CAD build for the part. Positions are in the model's coordinates, mm. A direction names the side the tool comes from. Round coordinates to 2 decimals unless told otherwise and drop trailing zeros. Order: outer loops, then holes, each group sorted by start corner. A loop starts at its lowest first (then second) coordinate and runs counter-clockwise, first axis right, second up. Notation, with made-up numbers: (26, 37) -> (47, 37) arc R32 cw to (47, 70) -> close; hole circle Ø9 at (-32.75, 1.5). An arc over 180 degrees is marked (long way). Return JSON: item names as keys, results as strings. Group by question number.
Q1. Which spindle directions (+Z, -Z, +X, -X, +Y, -Y) get a long thin tool onto all of the face, cutting with end or side? Do faces 4 (the flat face through (10, -0.574, 2)), 5 (the cylindrical face through (7.214, 13.802, 0.493)), 6 (the cylindrical face through (0.07, -2.96, 2.99)), 7 (the flat face through (-15, 22, 0)). Say none if no direction does.
Q2. Flat gauge pins, fed straight in: pin 1 (0.5 mm diameter, centred on y = 7, z = 3, fed in from +X); pin 2 (12.5 mm diameter, centred on x = 7, y = 3.5, fed in from +Z). Where does each tip first touch, or does it go through?
Q3. Cut at D-D (x = 9.5). Write the cut outline in (y, z).
Q4. Cut at A-A (x = 0). Write the cut outline in (y, z), then the cut area to 3 significant figures.
Q5. Mould opens along X. For faces 1 (the flat face through (11, 10, 1)), 2 (the cylindrical face through (3.34, -0.29, 2.99)), 3 (the cylindrical face through (0.57, 14.8, 1.23)) say: +X half, -X half, draft (parallel to the pull), parting line (faces both ways), or undercut.
Q6. Cut at C-C (z = 1.65). Count the separate pieces of the cut face and the enclosed holes in it, then the cut area to 3 significant figures.
Q7. Cut at B-B (y = 3). Write the cut outline in (x, z) (3 decimals), then the cut area to 3 significant figures.
Q8. Probe line 1 along Y through (x, z) = (0, 1.6); line 2 along Y through (x, z) = (8, 2.35); line 3 along X through (y, z) = (14.75, 0.4) (3 decimals). List the from-to ranges inside material, lowest first.
Autodesk Inventor part; units mm, degrees
ref_plane "YZ Plane" through (0, 0, 0) normal (1, 0, 0) x (0, 1, 0)
ref_plane "XZ Plane" through (0, 0, 0) normal (0, 1, 0) x (-1, 0, 0)
ref_plane "XY Plane" through (0, 0, 0) normal (0, 0, 1) x (1, 0, 0)
ref_plane "Work Plane1" through (0, 0, 0) normal (0, 0, 1) x (1, 0, 0)
sketch "Sketch1" plane through (0, 0, 0) normal (0, 0, 1) x (1, 0, 0)
  arc A0 (-3.651, 13.5937) -> (-4.7619, 15.391) centre (-4.2064, 14.4923) ccw
  arc A1 (-3.651, 13.5937) -> (-6.4477, 10.2643) centre (0, 7.6875) ccw
  arc A2 (-8.4097, 11.0483) -> (-6.4477, 10.2643) centre (-7.4287, 10.6563) ccw
  arc A3 (-4.7619, 15.391) -> (-8.4097, 11.0483) centre (0, 7.6875) ccw
  arc A4 (6.4477, 10.2643) -> (8.4097, 11.0483) centre (7.4287, 10.6563) ccw
  arc A5 (6.4477, 10.2643) -> (3.651, 13.5937) centre (0, 7.6875) ccw
  arc A6 (4.7619, 15.391) -> (3.651, 13.5937) centre (4.2064, 14.4923) ccw
  arc A7 (8.4097, 11.0483) -> (4.7619, 15.391) centre (0, 7.6875) ccw
  arc A8 (-6.4563, 5.1322) -> (-8.4209, 4.3547) centre (-7.4386, 4.7434) ccw
  arc A9 (-6.4563, 5.1322) -> (-3.651, 1.7813) centre (0, 7.6875) ccw
  arc A10 (-4.7619, -0.016) -> (-3.651, 1.7813) centre (-4.2064, 0.8827) ccw
  arc A11 (-8.4209, 4.3547) -> (-4.7619, -0.016) centre (0, 7.6875) ccw
  arc A12 (3.651, 1.7813) -> (4.7619, -0.016) centre (4.2064, 0.8827) ccw
  arc A13 (3.651, 1.7813) -> (6.4563, 5.1322) centre (0, 7.6875) ccw
  arc A14 (8.4209, 4.3547) -> (6.4563, 5.1322) centre (7.4386, 4.7434) ccw
  arc A15 (4.7619, -0.016) -> (8.4209, 4.3547) centre (0, 7.6875) ccw
  circle A16 centre (10.65, 7.6999) radius 1.15
  circle A17 centre (0, 15.6875) radius 1.0564
  circle A18 centre (0, -0.3125) radius 1.0564
  circle A19 centre (0, 7.6875) radius 5
  circle A20 centre (0, 7.6875) radius 13.7
  line L0 (-116.625, -11.1875) -> (15.375, -11.1875)
  line L1 (15.375, -11.1875) -> (15.375, -7.6875)
  line L2 (-116.625, -7.6875) -> (15.375, -7.6875)
  line L3 (-116.625, -11.1875) -> (-116.625, -7.6875)
  line L4 (15.375, -7.6875) -> (-15.375, -7.6875)
  line L5 (-15.375, -7.6875) -> (-15.375, 22.3125)
  line L6 (-15.375, 22.3125) -> (15.375, 22.3125)
  line L7 (15.375, 22.3125) -> (15.375, -7.6875)
  circle A21 centre (0, 7.6875) radius 14.375
  circle A22 centre (0, 7.6875) radius 5.2
  arc A23 (-3.4406, 13.2535) -> (-4.9722, 15.7312) centre (-4.2064, 14.4923) ccw
  arc A24 (-3.4406, 13.2535) -> (-6.0763, 10.1158) centre (0, 7.6875) ccw
  arc A25 (-8.7812, 11.1968) -> (-6.0763, 10.1158) centre (-7.4287, 10.6563) ccw
  arc A26 (-4.9722, 15.7312) -> (-8.7812, 11.1968) centre (0, 7.6875) ccw
  arc A27 (4.9722, 15.7312) -> (3.4406, 13.2535) centre (4.2064, 14.4923) ccw
  arc A28 (6.0763, 10.1158) -> (3.4406, 13.2535) centre (0, 7.6875) ccw
  arc A29 (6.0763, 10.1158) -> (8.7812, 11.1968) centre (7.4287, 10.6563) ccw
  arc A30 (8.7812, 11.1968) -> (4.9722, 15.7312) centre (0, 7.6875) ccw
  arc A31 (3.4406, 2.1215) -> (6.0844, 5.2794) centre (0, 7.6875) ccw
  arc A32 (3.4406, 2.1215) -> (4.9722, -0.3562) centre (4.2064, 0.8827) ccw
  arc A33 (4.9722, -0.3562) -> (8.7928, 4.2075) centre (0, 7.6875) ccw
  arc A34 (8.7928, 4.2075) -> (6.0844, 5.2794) centre (7.4386, 4.7434) ccw
  arc A35 (-6.0844, 5.2794) -> (-8.7928, 4.2075) centre (-7.4386, 4.7434) ccw
  arc A36 (-6.0844, 5.2794) -> (-3.4406, 2.1215) centre (0, 7.6875) ccw
  arc A37 (-4.9722, -0.3562) -> (-3.4406, 2.1215) centre (-4.2064, 0.8827) ccw
  arc A38 (-8.7928, 4.2075) -> (-4.9722, -0.3562) centre (0, 7.6875) ccw
  circle A39 centre (10.65, 7.6999) radius 1.55
  point P0 (0, 0)
  dimension "d0" = 30
  dimension "d1" = 15.375
  dimension "d2" = 15.375
  dimension "d3" = 0.2
  dimension "d4" = 0.4
  dimension "d5" = 0.4
  dimension "d6" = 0.4
  dimension "d7" = 0.4
  dimension "d8" = 0.4
extrude "Extrusion1" add sketch "Sketch1" along normal blind 1 contours A20 | L2 L5 L6 L7 | A21
sketch "Sketch2" plane through (0, 0, 1) normal (0, 0, 1) x (1, 0, 0)
  line L0 (15.375, 22.3125) -> (-15.375, 22.3125)
  line L1 (-15.375, 22.3125) -> (-15.375, -7.6875)
  line L2 (-15.375, -7.6875) -> (15.375, -7.6875)
  line L3 (15.375, -7.6875) -> (15.375, 22.3125)
  circle A0 centre (0, 15.6875) radius 1.0564
  circle A1 centre (0, -0.3125) radius 1.0564
  circle A2 centre (0, 7.6875) radius 5.2
  arc A3 (-3.4406, 13.2535) -> (-6.0763, 10.1158) centre (0, 7.6875) ccw
  arc A4 (-8.7812, 11.1968) -> (-6.0763, 10.1158) centre (-7.4287, 10.6563) ccw
  arc A5 (-4.9722, 15.7312) -> (-8.7812, 11.1968) centre (0, 7.6875) ccw
  arc A6 (-3.4406, 13.2535) -> (-4.9722, 15.7312) centre (-4.2064, 14.4923) ccw
  arc A7 (6.0763, 10.1158) -> (3.4406, 13.2535) centre (0, 7.6875) ccw
  arc A8 (4.9722, 15.7312) -> (3.4406, 13.2535) centre (4.2064, 14.4923) ccw
  arc A9 (8.7812, 11.1968) -> (4.9722, 15.7312) centre (0, 7.6875) ccw
  arc A10 (6.0763, 10.1158) -> (8.7812, 11.1968) centre (7.4287, 10.6563) ccw
  arc A11 (3.4406, 2.1215) -> (4.9722, -0.3562) centre (4.2064, 0.8827) ccw
  arc A12 (3.4406, 2.1215) -> (6.0844, 5.2794) centre (0, 7.6875) ccw
  arc A13 (8.7928, 4.2075) -> (6.0844, 5.2794) centre (7.4386, 4.7434) ccw
  arc A14 (4.9722, -0.3562) -> (8.7928, 4.2075) centre (0, 7.6875) ccw
  arc A15 (-6.0844, 5.2794) -> (-3.4406, 2.1215) centre (0, 7.6875) ccw
  arc A16 (-4.9722, -0.3562) -> (-3.4406, 2.1215) centre (-4.2064, 0.8827) ccw
  arc A17 (-8.7928, 4.2075) -> (-4.9722, -0.3562) centre (0, 7.6875) ccw
  arc A18 (-6.0844, 5.2794) -> (-8.7928, 4.2075) centre (-7.4386, 4.7434) ccw
  circle A19 centre (10.65, 7.6999) radius 1.55
  arc A20 (4.9722, 15.7312) -> (3.4406, 13.2535) centre (4.2064, 14.4923) ccw
  line L4 (4.2064, 15.9488) -> (15.375, 15.9488)
  line L5 (15.375, -7.6875) -> (15.375, 22.3125)
  line L6 (4.2064, -0.5738) -> (15.375, -0.5738)
  arc A21 (6.0763, 10.1158) -> (8.7812, 11.1968) centre (7.4287, 10.6563) ccw
  line L7 (6.0763, 10.1158) -> (6.0844, 5.2794)
  point P0 (0, 0)
extrude "Extrusion2" add sketch "Sketch2" along normal blind 1.5 contours L3 L4 A8 A7 L7 A12 A11 L6 L2 L1 L0
sketch "Sketch3" plane through (0, 0, 2.5) normal (0, 0, 1) x (1, 0, 0)
  line L0 (15.375, -7.6875) -> (15.375, -0.5738)
  line L1 (15.375, -0.5738) -> (4.2064, -0.5738)
  arc A0 (3.4406, 2.1215) -> (4.2064, -0.5738) centre (4.2064, 0.8827) ccw
  arc A1 (3.4406, 2.1215) -> (6.0844, 5.2794) centre (0, 7.6875) ccw
  line L2 (6.0844, 5.2794) -> (6.0763, 10.1158)
  arc A2 (6.0763, 10.1158) -> (3.4406, 13.2535) centre (0, 7.6875) ccw
  arc A3 (4.2064, 15.9488) -> (3.4406, 13.2535) centre (4.2064, 14.4923) ccw
  line L3 (4.2064, 15.9488) -> (15.375, 15.9488)
  line L4 (15.375, 15.9488) -> (15.375, 22.3125)
  line L5 (15.375, 22.3125) -> (-15.375, 22.3125)
  line L6 (-15.375, 22.3125) -> (-15.375, -7.6875)
  line L7 (-15.375, -7.6875) -> (15.375, -7.6875)
  circle A4 centre (0, 15.6875) radius 1.0564
  circle A5 centre (0, -0.3125) radius 1.0564
  arc A6 (-6.0844, 5.2794) -> (-8.7928, 4.2075) centre (-7.4386, 4.7434) ccw
  arc A7 (-6.0844, 5.2794) -> (-3.4406, 2.1215) centre (0, 7.6875) ccw
  arc A8 (-4.9722, -0.3562) -> (-3.4406, 2.1215) centre (-4.2064, 0.8827) ccw
  arc A9 (-8.7928, 4.2075) -> (-4.9722, -0.3562) centre (0, 7.6875) ccw
  arc A10 (-3.4406, 13.2535) -> (-4.9722, 15.7312) centre (-4.2064, 14.4923) ccw
  arc A11 (-3.4406, 13.2535) -> (-6.0763, 10.1158) centre (0, 7.6875) ccw
  arc A12 (-8.7812, 11.1968) -> (-6.0763, 10.1158) centre (-7.4287, 10.6563) ccw
  arc A13 (-4.9722, 15.7312) -> (-8.7812, 11.1968) centre (0, 7.6875) ccw
  circle A14 centre (0, 7.6875) radius 5.2
  circle A15 centre (0, 15.6875) radius 2.65
  circle A16 centre (0, -0.3125) radius 1.0564
  circle A17 centre (0, -0.3125) radius 2.65
  arc A18 (-2.4425, 10.6818) -> (-4.3563, 11.5819) centre (-5.3868, 6.906) ccw
  arc A19 (-4.3563, 11.5819) -> (-4.9119, 10.8525) centre (0, 7.6875) ccw
  arc A20 (-4.9119, 10.8525) -> (-3.5356, 9.2466) centre (-0.678, 13.0883) ccw
  arc A21 (-3.5356, 9.2466) -> (-3.736, 8.6743) centre (0, 7.6875) ccw
  arc A22 (-3.736, 8.6743) -> (-5.8134, 8.2775) centre (-3.8987, 3.889) ccw
  arc A23 (-5.8134, 8.2775) -> (-5.8341, 7.3609) centre (0, 7.6875) ccw
  arc A24 (-5.8341, 7.3609) -> (-3.7768, 6.8706) centre (-3.723, 11.6584) ccw
  arc A25 (-3.7768, 6.8706) -> (-3.6025, 6.2899) centre (0, 7.6875) ccw
  arc A26 (-3.6025, 6.2899) -> (-5.05, 4.7478) centre (-0.9214, 2.3228) ccw
  arc A27 (-5.05, 4.7478) -> (-4.5279, 3.994) centre (0, 7.6875) ccw
  arc A28 (-4.5279, 3.994) -> (-2.5753, 4.8067) centre (-5.346, 8.7117) ccw
  arc A29 (-2.5753, 4.8067) -> (-2.093, 4.4393) centre (0, 7.6875) ccw
  arc A30 (-2.093, 4.4393) -> (-2.3576, 2.341) centre (2.4078, 2.8058) ccw
  arc A31 (-2.3576, 2.341) -> (-1.4922, 2.038) centre (0, 7.6875) ccw
  arc A32 (-1.4922, 2.038) -> (-0.3902, 3.8431) centre (-4.927, 5.3738) ccw
  arc A33 (-0.3902, 3.8431) -> (0.216, 3.8294) centre (0, 7.6875) ccw
  arc A34 (0.216, 3.8294) -> (1.2353, 1.9763) centre (4.8174, 5.1534) ccw
  arc A35 (1.2353, 1.9763) -> (2.1135, 2.2398) centre (0, 7.6875) ccw
  arc A36 (2.1135, 2.2398) -> (1.944, 4.348) centre (-2.6261, 2.9196) ccw
  arc A37 (1.944, 4.348) -> (2.4425, 4.6932) centre (0, 7.6875) ccw
  arc A38 (2.4425, 4.6932) -> (4.3563, 3.7931) centre (5.3868, 8.469) ccw
  arc A39 (4.3563, 3.7931) -> (4.9119, 4.5225) centre (0, 7.6875) ccw
  arc A40 (4.9119, 4.5225) -> (3.5356, 6.1284) centre (0.678, 2.2867) ccw
  arc A41 (3.5356, 6.1284) -> (3.736, 6.7007) centre (0, 7.6875) ccw
  arc A42 (3.736, 6.7007) -> (5.8134, 7.0975) centre (3.8987, 11.486) ccw
  arc A43 (5.8134, 7.0975) -> (5.8341, 8.0141) centre (0, 7.6875) ccw
  arc A44 (5.8341, 8.0141) -> (3.7768, 8.5044) centre (3.723, 3.7166) ccw
  arc A45 (3.7768, 8.5044) -> (3.6025, 9.0851) centre (0, 7.6875) ccw
  arc A46 (3.6025, 9.0851) -> (5.05, 10.6272) centre (0.9214, 13.0522) ccw
  arc A47 (5.05, 10.6272) -> (4.5279, 11.381) centre (0, 7.6875) ccw
  arc A48 (4.5279, 11.381) -> (2.5753, 10.5683) centre (5.346, 6.6633) ccw
  arc A49 (2.5753, 10.5683) -> (2.093, 10.9357) centre (0, 7.6875) ccw
  arc A50 (2.093, 10.9357) -> (2.3576, 13.034) centre (-2.4078, 12.5692) ccw
  arc A51 (2.3576, 13.034) -> (1.4922, 13.337) centre (0, 7.6875) ccw
  arc A52 (1.4922, 13.337) -> (0.3902, 11.5319) centre (4.927, 10.0012) ccw
  arc A53 (0.3902, 11.5319) -> (-0.216, 11.5456) centre (0, 7.6875) ccw
  arc A54 (-0.216, 11.5456) -> (-1.2353, 13.3987) centre (-4.8174, 10.2216) ccw
  arc A55 (-1.2353, 13.3987) -> (-2.1135, 13.1352) centre (0, 7.6875) ccw
  arc A56 (-2.1135, 13.1352) -> (-1.944, 11.027) centre (2.6261, 12.4554) ccw
  arc A57 (-1.944, 11.027) -> (-2.4425, 10.6818) centre (0, 7.6875) ccw
  circle A58 centre (0, 7.6875) radius 5.8433
  circle A59 centre (0, 7.6875) radius 6.5436
  arc A60 (-3.4406, 13.2535) -> (-4.9722, 15.7312) centre (-4.2064, 14.4923) ccw
  line L8 (-2.9676, 15.2581) -> (-2.615, 15.2581)
  arc A61 (4.9722, 15.7312) -> (3.4406, 13.2535) centre (4.2064, 14.4923) ccw
  line L9 (2.9676, 15.2581) -> (2.615, 15.2581)
  arc A62 (3.4406, 2.1215) -> (4.9722, -0.3562) centre (4.2064, 0.8827) ccw
  line L10 (2.8055, 0.4846) -> (2.5273, 0.4846)
  arc A63 (-4.9722, -0.3562) -> (-3.4406, 2.1215) centre (-4.2064, 0.8827) ccw
  line L11 (-2.8055, 0.4846) -> (-2.5273, 0.4846)
  arc A64 (-8.7812, 11.1968) -> (-6.0763, 10.1158) centre (-7.4287, 10.6563) ccw
  line L12 (-7.7556, 9.237) -> (-7.7556, 6.165)
  point P0 (0, 0)
  point P1 (-6.0844, 5.2794)
  point P2 (-6.0763, 10.1158)
  point P3 (2.9676, 15.2581)
  dimension "d13" = 5.3
  dimension "d14" = 5.3
extrude "Extrusion3" add sketch "Sketch3" along normal blind 1 contours L7 L6 L5 L4 L3 A3 L9 A15 L8 A10 A13 A12 L12 A6 A9 A8 L11 A17 L10 A0 L1 L0
sketch "Sketch5" plane through (0, 0, 0) normal (0, 0, -1) x (-1, 0, 0)
  line L0 (-15.375, 22.3125) -> (15.375, 22.3125)
  line L1 (-15.375, -7.6875) -> (-15.375, 22.3125)
  line L2 (15.375, -7.6875) -> (-15.375, -7.6875)
  line L3 (15.375, 22.3125) -> (15.375, -7.6875)
  circle A0 centre (0, 15.6875) radius 1.0564
  circle A1 centre (0, -0.3125) radius 1.0564
  circle A2 centre (0, 7.6875) radius 5.2
  arc A3 (6.0763, 10.1158) -> (3.4406, 13.2535) centre (0, 7.6875) ccw
  arc A4 (4.9722, 15.7312) -> (3.4406, 13.2535) centre (4.2064, 14.4923) ccw
  arc A5 (8.7812, 11.1968) -> (4.9722, 15.7312) centre (0, 7.6875) ccw
  arc A6 (6.0763, 10.1158) -> (8.7812, 11.1968) centre (7.4287, 10.6563) ccw
  arc A7 (-3.4406, 13.2535) -> (-6.0763, 10.1158) centre (0, 7.6875) ccw
  arc A8 (-8.7812, 11.1968) -> (-6.0763, 10.1158) centre (-7.4287, 10.6563) ccw
  arc A9 (-4.9722, 15.7312) -> (-8.7812, 11.1968) centre (0, 7.6875) ccw
  arc A10 (-3.4406, 13.2535) -> (-4.9722, 15.7312) centre (-4.2064, 14.4923) ccw
  arc A11 (-4.9722, -0.3562) -> (-3.4406, 2.1215) centre (-4.2064, 0.8827) ccw
  arc A12 (-8.7928, 4.2075) -> (-4.9722, -0.3562) centre (0, 7.6875) ccw
  arc A13 (-6.0844, 5.2794) -> (-8.7928, 4.2075) centre (-7.4386, 4.7434) ccw
  arc A14 (-6.0844, 5.2794) -> (-3.4406, 2.1215) centre (0, 7.6875) ccw
  arc A15 (3.4406, 2.1215) -> (6.0844, 5.2794) centre (0, 7.6875) ccw
  arc A16 (8.7928, 4.2075) -> (6.0844, 5.2794) centre (7.4386, 4.7434) ccw
  arc A17 (4.9722, -0.3562) -> (8.7928, 4.2075) centre (0, 7.6875) ccw
  arc A18 (3.4406, 2.1215) -> (4.9722, -0.3562) centre (4.2064, 0.8827) ccw
  circle A19 centre (-10.65, 7.6999) radius 1.55
  circle A20 centre (-12.875, 19.8125) radius 2.5
  circle A21 centre (12.875, 19.8125) radius 2.5
  point P0 (0, 0)
  dimension "d26" = 5
  dimension "d27" = 5
  dimension "d28" = 2.5
  dimension "d29" = 2.5
  dimension "d30" = 2.5
  dimension "d31" = 2.5
hole "Hole2" at (12.875, 19.8125, 0) at (-12.875, 19.8125, 0) direction (0, 0, 1) diameter 3.1 end through all countersink diameter 5 countersink angle 90
equation "\"d2\" = d1"
equation "\"d28\" = 0.5 * d26"
equation "\"d29\" = 0.5 * d26"
equation "\"d30\" = 0.5 * d27"
equation "\"d31\" = 0.5 * d27"
properties part number "front_motur_holder" material "Nylon 6/6"
Solution:
{
 "1": {"face 4": "+Z, +X", "face 5": "+Z, -Z", "face 6": "+Z", "face 7": "-Z, +X, -X, +Y, -Y"},
 "2": {"pin 1": "stops at x = -7.76", "pin 2": "stops at z = 3.5"},
 "3": {"outline": "(-7.69, 0) -> (6.66, 0) -> (6.66, 1) -> (-0.57, 1) -> (-0.57, 3.5) -> (-7.69, 3.5) -> close; (8.74, 0) -> (22.31, 0) -> (22.31, 3.5) -> (15.95, 3.5) -> (15.95, 1) -> (8.74, 1) -> close"},
 "4": {"outline": "(-7.69, 0) -> (-1.37, 0) -> (-1.37, 2.5) -> (-2.96, 2.5) -> (-2.96, 3.5) -> (-7.69, 3.5) -> close; (0.74, 0) -> (2.49, 0) -> (2.49, 2.5) -> (0.74, 2.5) -> close; (12.89, 0) -> (14.63, 0) -> (14.63, 2.5) -> (12.89, 2.5) -> close; (16.74, 0) -> (22.31, 0) -> (22.31, 3.5) -> (18.34, 3.5) -> (18.34, 2.5) -> (16.74, 2.5) -> close", "area": "47.1 mm²"},
 "5": {"face 1": "draft", "face 2": "+X half", "face 3": "undercut"},
 "6": {"separate pieces": "1", "enclosed holes": "7", "area": "596 mm²"},
 "7": {"outline": "(-15.375, 0) -> (-8.213, 0) -> (-8.213, 3.5) -> (-15.375, 3.5) -> close; (-4.566, 0) -> (-2.251, 0) -> (-2.251, 2.5) -> (-4.566, 2.5) -> close; (2.251, 0) -> (4.566, 0) -> (4.566, 2.5) -> (2.251, 2.5) -> close; (8.213, 0) -> (15.375, 0) -> (15.375, 1) -> (8.213, 1) -> close", "area": "43.8 mm²"},
 "8": {"line 1": "y = -7.69 to -1.37, 0.74 to 2.49, 12.89 to 14.63, 16.74 to 22.31", "line 2": "y = -7.69 to -0.57, 15.95 to 22.31", "line 3": "x = -15.375 to -6.288, -2.773 to -0.487, 0.487 to 2.773, 6.289 to 15.375"}
}
